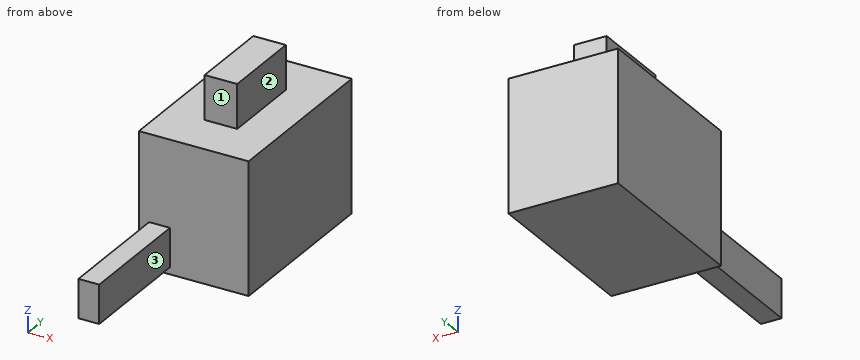
from build123d import *

# Parameters (mm, degrees)
F0_W     = 254
F0_H     = 406.4
F1_DEPTH = 304.8
F2_W     = 48.218414
F2_H     = 89.092545
F3_DEPTH = 279.4
F4_W     = 75.411438
F4_H     = 192.048072
F5_DEPTH = 101.6


with BuildPart() as f1:
    # F0 (on Top) → F1 (new body)
    with BuildSketch(Plane.XY):
        Rectangle(F0_W, F0_H)
    extrude(amount=F1_DEPTH)

    # F2 (on face) → F3 (join)
    with BuildSketch(Plane.XZ.offset(203.2)):
        with Locations((-79.117574, 60.734126)):
            Rectangle(F2_W, F2_H)
    extrude(amount=F3_DEPTH)

    # F4 (on face) → F5 (join)
    with BuildSketch(Plane.XY.offset(304.8)):
        Rectangle(F4_W, F4_H)
    extrude(amount=F5_DEPTH)


solid = f1.part
Check sheet for the modelled part. Datum: model origin and axes. Units: mm. Face numbers are marked on the shaded views. A direction names the side the tool comes from. Round coordinates to 2 decimals unless told otherwise and drop trailing zeros. Order: outer loops, then holes, each group sorted by start corner. A loop starts at its lowest first (then second) coordinate and runs counter-clockwise, first axis right, second up.
(1) Cross-section at D-D, the plane x = -46. Enter the section's corners in (y, z).
(2) Scan lines: probe 1 along Z at (x, y) = (116.5, 157); probe 2 along X at (y, z) = (-224, 85); probe 3 along Y at (x, z) = (-51, 24.5). Record each from-to range of solid material in increasing order.
(3) Cross-section at A-A, the plane x = -85.5. Enter the section's corners in (y, z), and give its area (3 significant figures).
(4) Go/stop test with flat-tipped pins: P1, Ø6, axis at x = 84.5, z = 240.5, coming from the -Y side; P2, Ø24, axis at x = -74, y = -365, coming from the -Z side; P3, Ø4, axis at y = -87, z = 362.5, coming from the +X side. Record where each tip stops, or that it passes through.
(5) Access from +Z, -Z, +X, -X, +Y, -Y to the whole of each face (thin tool, end or side, straight path). Record for the marked faces 1, 2 and 3.
(6) Cross-section at C-C, the plane z = 294.5. Enter the section's corners in (x, y).
(7) Cross-section at B-B, the plane y = -49.5. Enter the section's corners in (x, z).
Check sheet entries:
1. outline: (-203.2, 0) - (203.2, 0) - (203.2, 304.8) - (-203.2, 304.8) - close
2. probe 1: z = 0 to 304.8
2. probe 2: x = -103.23 to -55.01
2. probe 3: y = -203.2 to 203.2
3. outline: (-482.6, 16.19) - (-203.2, 16.19) - (-203.2, 0) - (203.2, 0) - (203.2, 304.8) - (-203.2, 304.8) - (-203.2, 105.28) - (-482.6, 105.28) - close
3. area: 149,000 mm2
4. P1: stops at y = -203.2
4. P2: stops at z = 16.19
4. P3: stops at x = 37.71
5. face 1: +Z, +X, -X, -Y
5. face 2: +Z, +X, +Y, -Y
5. face 3: +Z, -Z, +X, -Y
6. outline: (-127, -203.2) - (127, -203.2) - (127, 203.2) - (-127, 203.2) - close
7. outline: (-127, 0) - (127, 0) - (127, 304.8) - (37.71, 304.8) - (37.71, 406.4) - (-37.71, 406.4) - (-37.71, 304.8) - (-127, 304.8) - close
